Source: three-view drawing plus pictorial views. Frame: mm from the lowest corner of the part. Give positions to 0.01 mm unless a question says otherwise; leave off trailing zeros. Order: outer loops, then holes, each group sorted by start corner. A loop starts at its lowest first (then second) coordinate and runs counter-clockwise, first axis right, second up. Notation, with made-up numbers: (64, 63.25) -> (103, 63.25) arc R13 cw to (103, 67.25) -> close; hole circle Ø5 at (73, 57). An arc over 180 degrees is marked (long way). Answer in a Markdown table with one row per item.
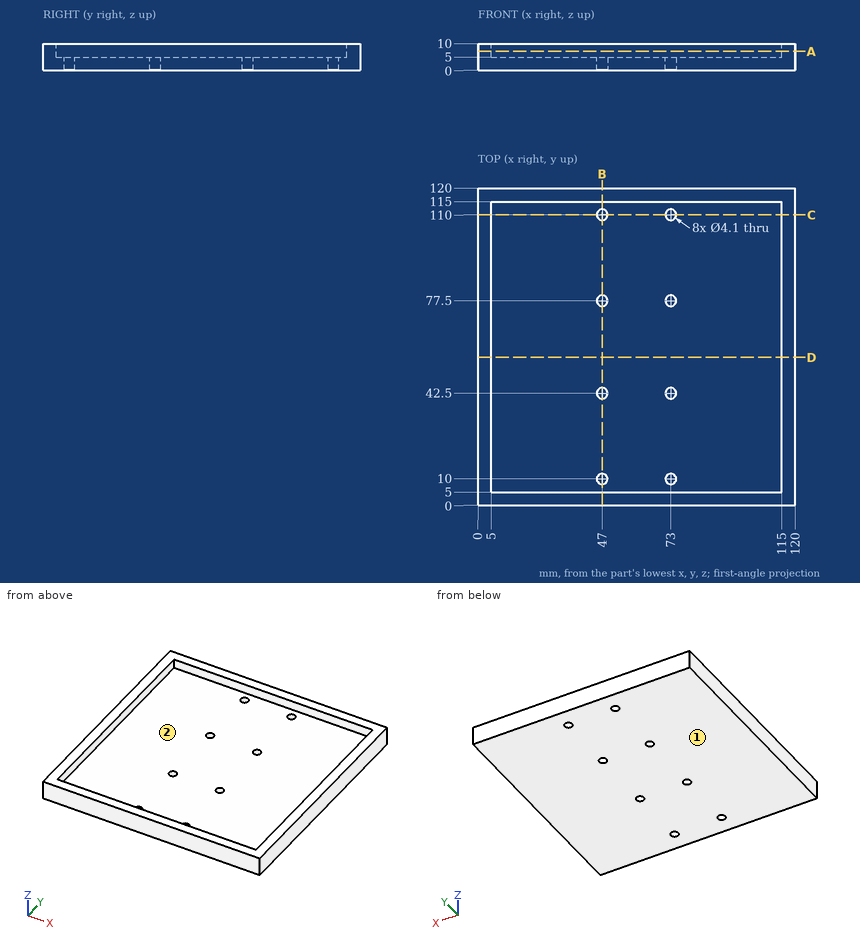
(1) Section query D-D (y = 56). Return the cut outline in (x, z).
A:
| item | result |
|---|---|
| outline | (0, 0) -> (120, 0) -> (120, 10) -> (115, 10) -> (115, 5) -> (5, 5) -> (5, 10) -> (0, 10) -> close |
(2) Pull-direction query (X, two-part tool) for the marked faces 1 and 2; classes: +X half, -X half, draft (parallel to the pull), parting line (faces both ways), or undercut.
A:
| item | result |
|---|---|
| face 1 | draft |
| face 2 | undercut |
(3) Section query A-A (z = 7.25). Return the cut outline in (x, y), plus the area to 3 significant figures.
A:
| item | result |
|---|---|
| outline | (0, 0) -> (120, 0) -> (120, 120) -> (0, 120) -> close; hole (5, 5) -> (115, 5) -> (115, 115) -> (5, 115) -> close |
| area | 2,300 mm^2 |
(4) Ray query, probe 1 along X at (y, z) = (110, 1.2); probe 2 along Y at (x, z) = (73, 1.45); probe 3 along X at (y, z) = (13, 6.75). Return the intervals inside material, ascending.
A:
| item | result |
|---|---|
| probe 1 | x = 0 to 44.95, 49.05 to 70.95, 75.05 to 120 |
| probe 2 | y = 0 to 7.95, 12.05 to 40.45, 44.55 to 75.45, 79.55 to 107.95, 112.05 to 120 |
| probe 3 | x = 0 to 5, 115 to 120 |
(5) Section query B-B (x = 47). Return the cut outline in (y, z), plus the area to 3 significant figures.
A:
| item | result |
|---|---|
| outline | (0, 0) -> (7.95, 0) -> (7.95, 5) -> (5, 5) -> (5, 10) -> (0, 10) -> close; (12.05, 0) -> (40.45, 0) -> (40.45, 5) -> (12.05, 5) -> close; (44.55, 0) -> (75.45, 0) -> (75.45, 5) -> (44.55, 5) -> close; (79.55, 0) -> (107.95, 0) -> (107.95, 5) -> (79.55, 5) -> close; (112.05, 0) -> (120, 0) -> (120, 10) -> (115, 10) -> (115, 5) -> (112.05, 5) -> close |
| area | 568 mm^2 |
(6) First-contact query: pin 1 Ø12 at (x, y) = (48.5, 85) entering from +Z. Flat tip, straight axial feed; report the tip coordinate or a pass-through.
A:
| item | result |
|---|---|
| pin 1 | stops at z = 5 |
(7) Section query C-C (y = 110). Return the cut outline in (x, z), plus the area to 3 significant figures.
A:
| item | result |
|---|---|
| outline | (0, 0) -> (44.95, 0) -> (44.95, 5) -> (5, 5) -> (5, 10) -> (0, 10) -> close; (49.05, 0) -> (70.95, 0) -> (70.95, 5) -> (49.05, 5) -> close; (75.05, 0) -> (120, 0) -> (120, 10) -> (115, 10) -> (115, 5) -> (75.05, 5) -> close |
| area | 609 mm^2 |
